Read the model definition and answer for the solid it produces. Units are mm, in the model's axes. Face numbers are marked on the shaded views. A direction names the side the tool comes from. Round coordinates to 2 decimals unless told otherwise and drop trailing zeros. Write each loop counter-clockwise with the first axis right and the second up, starting at its lowest first coordinate (ties: lowest second). Pieces come first, ordered by that corner, then holes.
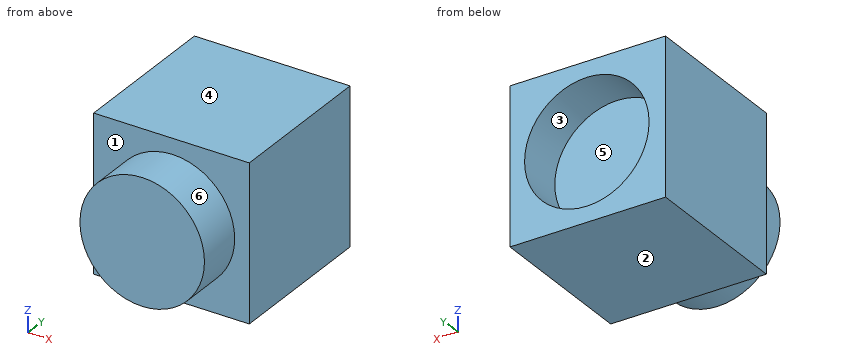
from build123d import *

# Parameters (mm, degrees)
F0_W     = 254
F0_H     = 254
F1_DEPTH = 254
F2_R     = 101.6
F3_DEPTH = 76.2
F4_R     = 101.6
F5_DEPTH = 76.2


with BuildPart() as f1:
    # F0 (on Top) → F1 (new body)
    with BuildSketch(Plane.XY):
        with Locations((-1.528222, -2.116666)):
            Rectangle(F0_W, F0_H)
    extrude(amount=F1_DEPTH)

    # F2 (on face) → F3 (join)
    with BuildSketch(Plane.XZ.offset(129.116666)):
        with Locations((0, 127)):
            Circle(F2_R)
    extrude(amount=F3_DEPTH)

    # F4 (on face) → F5 (cut)
    with BuildSketch(Plane(origin=(0, 124.883334, 0), x_dir=(-1, 0, 0), z_dir=(0, 1, 0))):
        with Locations((0, 127)):
            Circle(F4_R)
    extrude(amount=-F5_DEPTH, mode=Mode.SUBTRACT)


solid = f1.part
Q1. Straight lines are drawn through the part: probe 1 along Z at (x, y) = (0, 96); probe 2 along X at (y, z) = (90, 123.5); probe 3 along Y at (x, z) = (-11, 154.5). For each, find the intervals that lie inside material, in ascending order.
Verdict:
probe 1: z = 0 to 25.4, 228.6 to 254
probe 2: x = -128.53 to -101.54, 101.54 to 125.47
probe 3: y = -205.32 to 48.68
Q2. Determine the mould class of the marked faces 1, 2 and 3 for opening direction Z: pulls with the +Z half, pulls with the -Z half, needs draft (parallel to the pull), parting line crosses it, or undercut.
Verdict:
face 1: needs draft
face 2: pulls with the -Z half
face 3: undercut
Q3. Section A-A (x = 0) is taken. Determine the outline of the cut face in (y, z), then the cut area to 3 significant figures.
Verdict:
outline: (-205.32, 25.4) - (-129.12, 25.4) - (-129.12, 0) - (124.88, 0) - (124.88, 25.4) - (48.68, 25.4) - (48.68, 228.6) - (124.88, 228.6) - (124.88, 254) - (-129.12, 254) - (-129.12, 228.6) - (-205.32, 228.6) - close
area: 64,500 mm2
Q4. Section B-B (z = 133.5) is taken. Determine the outline of the cut face in (x, y), then the cut area to 3 significant figures.
Verdict:
outline: (-128.53, -129.12) - (-101.39, -129.12) - (-101.39, -205.32) - (101.39, -205.32) - (101.39, -129.12) - (125.47, -129.12) - (125.47, 124.88) - (101.39, 124.88) - (101.39, 48.68) - (-101.39, 48.68) - (-101.39, 124.88) - (-128.53, 124.88) - close
area: 64,500 mm2
Q5. Which of the six approach directions +Z, -Z, +X, -X, +Y, -Y give full straight-line access (tool end or side, diameter ignored) to the marked faces 4, 5 and 6?
Verdict:
face 4: +Z, +X, -X, +Y, -Y
face 5: +Y
face 6: -Y
Q6. Flat-ended cylindrical pins translate along their axes: pin 1 Ø3 at (x, y) = (35, -32) entering from -Z; pin 2 Ø8 at (x, y) = (-10.5, -150) entering from -Z; pin 3 Ø5 at (x, z) = (-55, 37.5) entering from -Y; pin 4 Ø1 at (y, z) = (-164, 132.5) entering from -X. Find the tip coordinate at first contact, or state that the pin passes through.
Verdict:
pin 1: stops at z = 0
pin 2: stops at z = 25.61
pin 3: stops at y = -129.12
pin 4: stops at x = -101.48
